Part model, mm, in its own coordinate system. Face numbers are marked on the shaded views. Coordinates: 2 decimals unless noted, no trailing zeros. Write each loop counter-clockwise with the first axis right and the second up, starting at its lowest first coordinate (ties: lowest second). Pieces come first, ordered by that corner, then holes. Notation, with made-up numbers: (59, 5) -> (72, 5) arc R19 cw to (72, 27) -> close; hole circle Ø5 at (-5.75, 38). An arc over 180 degrees is marked (long way). Write item = value, one per line.
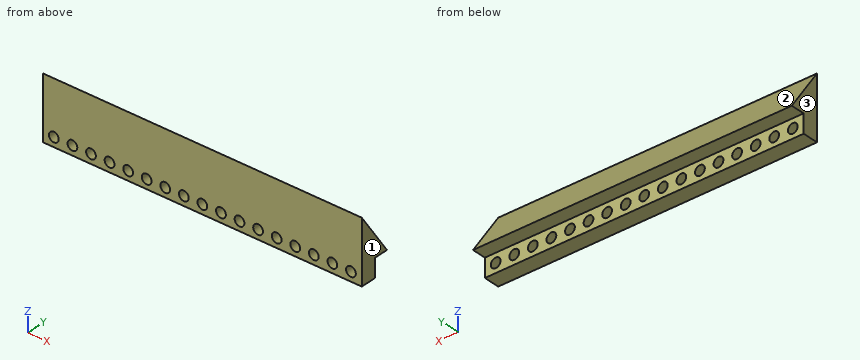
Autodesk Inventor part; units mm, degrees
ref_plane "Work Plane1" through (87.3566, 19.05, 5.6027) normal (0, -0.9396926, -0.3420201) x (-1, 0, 0)
ref_plane "Work Plane2" through (-79.1934, 19.05, 5.6027) normal (0, 1, 0) x (1, 0, 0)
ref_plane "YZ Plane" through (0, 0, 0) normal (1, 0, 0) x (0, 1, 0)
sketch "Sketch1" plane through (0, 0, 0) normal (0, 1, 0) x (-1, 0, 0)
  line L0 (60.1434, 43.7027) -> (-87.3566, 43.7027)
  line L1 (-87.3566, 43.7027) -> (-87.3566, 5.6027)
  line L2 (-87.3566, 5.6027) -> (60.1434, 5.6027)
  line L3 (60.1434, 5.6027) -> (60.1434, 43.7027)
  point P0 (0, 0)
  dimension "d0" = 147.5
  dimension "d1" = 38.1
extrude "Extrusion1" add sketch "Sketch1" along normal blind 19.05
ref_plane "Work Plane1" through (87.3566, 19.05, 5.6027) normal (0, -0.9396926, -0.3420201) x (-1, 0, 0)
sketch "Sketch2" plane through (87.3566, 19.05, 5.6027) normal (0, -0.9396926, -0.3420201) x (-1, 0, 0)
  line L0 (147.5, -42.3178) -> (147.5, -35.8023) construction
  line L1 (0, -35.8023) -> (0, 0) construction
  line L2 (147.5, -40.4915) -> (0, -40.4915)
  line L3 (0, -40.4915) -> (0, 0)
  line L4 (0, 0) -> (147.5, 0)
  line L5 (147.5, 0) -> (147.5, -40.4915)
  point P0 (87.3566, -1.2507)
extrude "Extrusion2" add sketch "Sketch2" against normal blind 19.05
sketch "Sketch3" plane through (87.3566, 36.9511, 12.1182) normal (0, 0.9396926, 0.3420201) x (1, 0, 0)
  line L0 (0, -40.4915) -> (-147.5, -40.4915) construction
  line L1 (0, -6.5155) -> (0, 0) construction
  line L2 (-147.5, -40.4915) -> (0, -40.4915)
  line L3 (0, -40.4915) -> (0, 0)
  line L4 (0, 0) -> (-147.5, 0)
  line L5 (-147.5, 0) -> (-147.5, -40.4915)
  point P0 (-87.3566, -1.2507)
extrude "Extrusion3" cut sketch "Sketch3" against normal blind 19.05
ref_plane "Work Plane2" through (-79.1934, 19.05, 5.6027) normal (0, 1, 0) x (1, 0, 0)
fillet "Fillet2" radius 3.175 5 edges at (13.6066, 5.3397, 43.7027) (13.6066, 0, 43.7027) (-60.1434, 0, 24.6527) (13.6066, 0, 5.6027) (87.3566, 0, 24.6527)
fillet "Fillet3" radius 3.175 1 edges at (13.6066, 19.0479, 5.6027)
sketch "Sketch12" plane through (87.3566, 3.175, 43.7027) normal (1, 0, 0) x (0, 0, -1)
  line L0 (38.121, 6.8749) -> (30.121, 6.8749)
  line L1 (30.121, 6.8749) -> (30.121, 14.8749)
  line L2 (30.121, 14.8749) -> (38.121, 14.8749)
  line L3 (38.121, 14.8749) -> (38.121, 6.8749)
  dimension "d36" = 8
  dimension "d37" = 8
extrude "Extrusion9" cut sketch "Sketch12" against normal through all
sketch "Sketch13" plane through (87.3566, 10.0499, 13.5817) normal (0, 1, 0) x (1, 0, 0)
  line L0 (-73.75, 7.979) -> (-73.75, -0.1527)
  circle A0 centre (-73.75, 3.9895) radius 2.1
  circle A1 centre (-81.75, 3.9895) radius 2.1
  circle A2 centre (-89.75, 3.9895) radius 2.1
  circle A3 centre (-97.75, 3.9895) radius 2.1
  circle A4 centre (-105.75, 3.9895) radius 2.1
  circle A5 centre (-113.75, 3.9895) radius 2.1
  circle A6 centre (-121.75, 3.9895) radius 2.1
  circle A7 centre (-129.75, 3.9895) radius 2.1
  circle A8 centre (-137.75, 3.9895) radius 2.1
  circle A9 centre (-65.75, 3.9895) radius 2.1
  circle A10 centre (-57.75, 3.9895) radius 2.1
  circle A11 centre (-49.75, 3.9895) radius 2.1
  circle A12 centre (-41.75, 3.9895) radius 2.1
  circle A13 centre (-33.75, 3.9895) radius 2.1
  circle A14 centre (-25.75, 3.9895) radius 2.1
  circle A15 centre (-17.75, 3.9895) radius 2.1
  circle A16 centre (-9.75, 3.9895) radius 2.1
extrude "Extrusion10" cut sketch "Sketch13" against normal through all
sketch "Sketch14" plane through (87.3566, 3.175, 43.7027) normal (1, 0, 0) x (0, 0, -1)
  line L0 (-30.4844, 21.6462) -> (52.8728, 21.6462)
  line L1 (52.8728, 21.6462) -> (52.8728, -12.2101)
  line L2 (52.8728, -12.2101) -> (-30.4844, -12.2101)
  line L3 (-30.4844, -12.2101) -> (-30.4844, 21.6462)
  point P0 (43.7027, -3.175)
extrude "Extrusion11" cut sketch "Sketch14" against normal blind 5.08
sketch "Sketch15" plane through (-60.1434, 3.175, 43.7027) normal (-1, 0, 0) x (0, 0, 1)
  line L0 (33.6252, 94.5491) -> (-79.5372, 94.5491)
  line L1 (-79.5372, 94.5491) -> (-79.5372, -54.7848)
  line L2 (-79.5372, -54.7848) -> (33.6252, -54.7848)
  line L3 (33.6252, -54.7848) -> (33.6252, 94.5491)
  point P0 (-43.7027, -3.175)
extrude "Extrusion12" cut sketch "Sketch15" against normal blind 5.08
sketch "Sketch16" plane through (82.2766, 3.175, 43.7027) normal (1, 0, 0) x (0, 0, -1)
  arc A0 (34.925, -3.175) -> (38.1, 0) centre (34.925, 0) ccw construction
  line L0 (-8.1127, -3.175) -> (38.1, -3.175)
  line L1 (38.1, -3.175) -> (38.1, 0)
  line L2 (38.1, 0) -> (-8.1127, 0)
  line L3 (-8.1127, 0) -> (-8.1127, -3.175)
  line L4 (0, 1.4623) -> (0, 0) construction
  line L5 (30.121, 12.9709) -> (11.0545, 0)
  line L6 (11.2811, 0) -> (-2.3132, 0)
  line L7 (-2.3132, 0) -> (0.9299, 12.0527)
  line L8 (0.0505, 2.0261) -> (30.121, 12.9709) construction
  line L9 (0.9299, 12.0527) -> (30.121, 12.9709)
  point P0 (43.7027, -3.175)
  point P1 (0, 0.7312)
extrude "Extrusion14" cut sketch "Sketch16" against normal through all
sketch "Sketch17" plane through (82.2766, 3.175, 43.7027) normal (1, 0, 0) x (0, 0, -1)
  line L0 (30.121, 12.9709) -> (11.0545, 0) construction
  line L1 (11.0545, 0) -> (38.1, 0) construction
  line L2 (38.1, 6.8749) -> (38.1, 0) construction
  line L3 (30.121, 6.8749) -> (38.1, 6.8749) construction
  line L4 (30.121, 12.9709) -> (30.121, 6.8749) construction
  point P0 (43.7027, -3.175)
properties part number "Ramp version 1"
Q1. Saw through at B-B on y = 5.25. Count the separate pieces of the cut face and the enclosed holes in it, and give its area (3 significant figures).
Model answer:
separate_pieces = 1
enclosed_holes = 17
area = 3,060 mm²
Q2. Saw through at C-C on x = 9. Give the cut face in (y, z) (3 decimals), and give its area (3 significant figures).
Model answer:
outline = (3.175, 5.603) -> (10.05, 5.603) -> (10.05, 13.582) -> (16.144, 13.582) -> (16.141, 13.589) -> (3.175, 32.648) -> close
area = 179 mm²
Q3. Saw through at D-D on z = 23. Give the cut face in (x, y) (3 decimals).
Model answer:
outline = (-55.063, 3.175) -> (82.277, 3.175) -> (82.277, 9.739) -> (-55.063, 9.739) -> close
Q4. Mould opens along X. For the marked faces 1, 2 and 3 say: released by +X, released by -X, zero draft, split by the parting line, or undercut.
Model answer:
face_1 = released by +X
face_2 = zero draft
face_3 = released by -X
Q5. Probe line 1 (Y direction, x = 8, z = 9.75) (3 decimals); line 2 (Z direction, x = 7, y = 4.75); line 3 (Z direction, x = 54, y = 7.5). List the from-to ranges inside material, lowest first. Write a range as from..to.
Model answer:
line_1 = 3.175..10.05
line_2 = 5.6..8.02, 11.16..30.33
line_3 = 5.6..7.53, 11.66..26.29
Q6. Pin check, flat tips, straight feed: pin 1 (9 mm diameter, centred on x = -8, z = 8, fed in from +Y); pin 2 (4 mm diameter, centred on x = -50.39, z = 9.59, fed in from +Y); pin 3 (6 mm diameter, centred on x = 30.5, z = 26.5, fed in from +Y); pin 4 (2 mm diameter, centred on x = -12.5, y = 13, fed in from -Z). Stop position of each tip, or through.
Model answer:
pin_1 = 10.05
pin_2 = through
pin_3 = 9.4
pin_4 = 13.58
Q7. Saw through at A-A on x = 38. Give the cut face in (y, z) (3 decimals), and give its area (3 significant figures).
Model answer:
outline = (3.175, 5.603) -> (10.05, 5.603) -> (10.05, 7.529) -> (3.175, 7.529) -> close; (3.175, 11.655) -> (10.05, 11.655) -> (10.05, 13.582) -> (16.144, 13.582) -> (16.141, 13.589) -> (3.175, 32.648) -> close
area = 150 mm²
